```python
from build123d import *

# Parameters (mm, degrees)
F1_DEPTH = 6.35


with BuildPart() as f1:
    # F0 (on Front) → F1 (new body)
    with BuildSketch(Plane.XZ):
        with BuildLine():
            ThreePointArc((15.875, 31.75), (10.454936, 33.995064), (12.7, 28.575))
            ThreePointArc((12.7, 28.575), (14.945064, 29.504936), (15.875, 31.75))
        make_face()
        Polygon((0, 12.7), (0, 0), (12.7, 0), (25.4, 0), (25.4, 12.7), (22.86, 25.4), (22.86, 38.1), (2.54, 38.1), (2.54, 25.4), align=None)
        with BuildLine():
            ThreePointArc((15.875, 31.75), (14.945064, 29.504936), (12.7, 28.575))
            ThreePointArc((12.7, 28.575), (10.454936, 33.995064), (15.875, 31.75))
        make_face(mode=Mode.SUBTRACT)
    extrude(amount=F1_DEPTH)


solid = f1.part
```
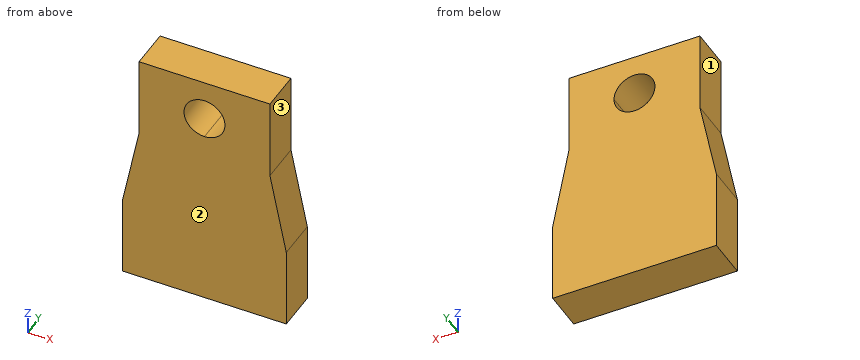
The listing builds one solid part. Answer for the finished solid, in the listing's coordinates (mm). Face numbers are marked on the shaded views. A direction names the side the tool comes from. Give positions to 0.01 mm unless a question says otherwise; leave off trailing zeros. Order: outer loops, then holes, each group sorted by start corner. A loop starts at its lowest first (then second) coordinate and runs counter-clockwise, first axis right, second up. Notation, with made-up numbers: (21.5, 30) - (65.5, 30) arc R35 cw to (65.5, 69) - close; hole circle Ø6 at (83, -4). An arc over 180 degrees is marked (long way). Answer in a Markdown table with one row per item. Add a question column.
Q1. Find the intervals of material crossed by line 1 along X through (y, z) = (-2.5, 31.75) (3 decimals); line 2 along Z through (x, y) = (12.7, -4.75) (3 decimals); line 3 along Z through (x, y) = (14.25, -2), in increasing order. Write a range as [from, to].
Q2. The part is cut by section B-B (x = 13.5). Determine the outline of the cut face in (y, z).
Q3. The part is cut by section C-C (z = 16). Determine the outline of the cut face in (x, y), then the cut area to 3 significant figures.
Q4. The part is cut by section A-A (z = 34). Determine the outline of the cut face in (x, y), then the cut area to 3 significant figures.
Q5. The part is cut by section D-D (x = 2). Determine the outline of the cut face in (y, z), then the cut area to 3 significant figures.
Q6. Given P1, Ø1.9, axis at y = -4, z = 29.5, coming from the -X side; P2, Ø4, axis at x = 12.7, z = 31.75, coming from the -Y side; P3, Ø1, axis at y = -2.5, z = 18, coming from the -X side, each flat-ended and moving along its own axis, determine where each tip first touches the part or whether it passes through.
Q7. Which of the six approach directions +Z, -Z, +X, -X, +Y, -Y give full straight-line access (tool end or side, diameter ignored) to the marked faces 1, 2 and 3?
Determined:
| question | item | result |
|---|---|---|
| 1 | line 1 | x = [2.54, 9.525], [15.875, 22.86] |
| 1 | line 2 | z = [0, 28.575], [34.925, 38.1] |
| 1 | line 3 | z = [0, 28.98], [34.52, 38.1] |
| 2 | outline | (-6.35, 0) - (0, 0) - (0, 28.68) - (-6.35, 28.68) - close; (-6.35, 34.82) - (0, 34.82) - (0, 38.1) - (-6.35, 38.1) - close |
| 3 | outline | (0.66, -6.35) - (24.74, -6.35) - (24.74, 0) - (0.66, 0) - close |
| 3 | area | 153 mm² |
| 4 | outline | (2.54, -6.35) - (10.46, -6.35) - (10.46, 0) - (2.54, 0) - close; (14.94, -6.35) - (22.86, -6.35) - (22.86, 0) - (14.94, 0) - close |
| 4 | area | 101 mm² |
| 5 | outline | (-6.35, 0) - (0, 0) - (0, 22.7) - (-6.35, 22.7) - close |
| 5 | area | 144 mm² |
| 6 | P1 | stops at x = 2.54 |
| 6 | P2 | passes through |
| 6 | P3 | stops at x = 0.96 |
| 7 | face 1 | +Z, -X, +Y, -Y |
| 7 | face 2 | +Z, -Z, +X, -X, -Y |
| 7 | face 3 | +Z, +X, +Y, -Y |
